CAD build for the part. Positions are in the model's coordinates, mm. Give positions to 0.01 mm unless a question says otherwise; leave off trailing zeros. Write each loop counter-clockwise with the first axis right and the second up, starting at its lowest first coordinate (ties: lowest second). Pieces come first, ordered by that corner, then holes. Notation, with made-up numbers: (85, -16) - (97, -16) arc R28 cw to (97, 16) - close; hole circle Ø2 at (61.25, 9.25). An arc over 180 degrees is marked (long way). Put each result on its own line as item: value. Start each with the question number.
1. Wall check: line 1 (X direction, y = -19, z = 4.8); line 2 (Y direction, x = -24.5, z = 1.05); line 3 (Y direction, x = 24.5, z = 2.15). Give the ranges that are in metal, low to high.
2. Mould opens along Y. For faces 1 (the flat face through (0, -24.892, 3)), 2 (the cylindrical face through (-25.874, -21.863, 2.576)), 3 (the flat face through (0, 6, 5.08)) say: +Y half, -Y half, draft (parallel to the pull), parting line (faces both ways), or undercut.
3. Cut at B-B on x = -14.5. List the corners of the cut face in (y, z).
4. Cut at A-A on z = 3. List the corners of the cut face in (x, y).
5. Cut at C-C on y = 22.5. List the corners of the cut face in (x, z).
6. Drop a flat-ended pin along its axis: pin 1 (1 mm diameter, centred on y = 22, z = 1.5, fed in from -X). Give the stop position or say it passes through.
from build123d import *

# Parameters (mm, degrees)
SKETCH1_R           = 35.56
BOSS_EXTRUDE1_DEPTH = 5.08
CUT_EXTRUDE1_DEPTH  = 51.545361805
SKETCH7_R           = 2.032
CUT_EXTRUDE2_DEPTH  = 51.545361805


with BuildPart() as part:
    # Sketch1 → Boss-Extrude1 (new body)
    with BuildSketch(Plane.XY):
        Circle(SKETCH1_R)
    extrude(amount=BOSS_EXTRUDE1_DEPTH)

    # Sketch2 → Cut-Extrude1 (cut, through all)
    with BuildSketch(Plane.XY.offset(5.08)):
        Polygon((0, -35.56), (-36.256055522, -35.56), (-36.256055522, -24.892), (33.75035888, -24.892), (33.75035888, -35.56), align=None)
    extrude(amount=-CUT_EXTRUDE1_DEPTH, mode=Mode.SUBTRACT)

    # Sketch7 → Cut-Extrude2 (cut, through all)
    with BuildSketch(Plane.XY.offset(5.08)):
        with Locations((-24.261099887, -20.626476503)):
            Circle(SKETCH7_R)
        with Locations((-7.471969114, 29.665523497)):
            Circle(SKETCH7_R)
        with Locations((25.522900113, -7.952823738)):
            Circle(SKETCH7_R)
    extrude(amount=-CUT_EXTRUDE2_DEPTH, mode=Mode.SUBTRACT)


solid = part.part
Report:
1. line 1: x = -30.06 to -25.48, -23.04 to 30.06
1. line 2: y = -24.89 to -22.64, -18.61 to 25.77
1. line 3: y = -24.89 to -9.71, -6.2 to 25.77
2. face 1: -Y half
2. face 2: undercut
2. face 3: draft
3. outline: (-24.89, 0) - (32.47, 0) - (32.47, 5.08) - (-24.89, 5.08) - close
4. outline: (-25.39, -24.89) - (25.39, -24.89) arc R35.56 ccw (long way) to start; hole circle Ø4.06 at (-24.26, -20.63); hole circle Ø4.06 at (-7.47, 29.67); hole circle Ø4.06 at (25.52, -7.95)
5. outline: (-27.54, 0) - (27.54, 0) - (27.54, 5.08) - (-27.54, 5.08) - close
6. pin 1: stops at x = -28.32
